Read the model definition and answer for the solid it produces. Units are mm, in the model's axes. Round coordinates to 2 decimals unless told otherwise and drop trailing zeros. Write each loop counter-clockwise with the first axis right and the second up, starting at its lowest first coordinate (ties: lowest second). Pieces come first, ordered by that corner, then holes. Notation, with made-up numbers: (50, -33) -> (106, -33) arc R8 cw to (106, -20) -> close; hole circle Ø7 at (24.25, 81). An arc over 180 degrees is marked (long way). Return JSON: item names as keys, results as strings. Group by question number.
(1) Straight lines are drawn through the part: line 1 (X direction, y = 16, z = 6); line 2 (Z direction, x = 29, y = 16.25); line 3 (Z direction, x = 6.5, y = 4). For each, find the intervals that lie inside material, in ascending order.
(2) A cutting plane is placed at D-D on y = 15.5. Give the vertices of the cut face in (x, z).
(3) The mould has two halves that part along Y. Classify faces 1 (the cylindrical face through (14.05, 13.7, 14.79)), 2 (the cylindrical face through (30.908, 11.154, 23.399)), 3 (the flat face through (17, 0, 15)): released by +Y, released by -Y, zero draft, split by the parting line, or undercut.
(4) A cutting plane is placed at A-A on x = 5. Give the vertices of the cut face in (y, z).
(5) A cutting plane is placed at C-C on x = 17. Give the vertices of the cut face in (y, z), then the cut area to 3 significant figures.
(6) A cutting plane is placed at B-B on z = 6. Give the vertices of the cut face in (x, y).
```python
from build123d import *

# Parameters (mm, degrees)
SKETCH1_W           = 34
SKETCH1_H           = 22
SKETCH1_R           = 4
BOSS_EXTRUDE1_DEPTH = 30
SKETCH2_R           = 2
CUT_EXTRUDE1_DEPTH  = 23


with BuildPart() as part:
    # Sketch1 → Boss-Extrude1 (new body)
    with BuildSketch(Plane.XY):
        with Locations((17, 11)):
            Rectangle(SKETCH1_W, SKETCH1_H)
        with Locations((17, 11)):
            Circle(SKETCH1_R, mode=Mode.SUBTRACT)
    extrude(amount=BOSS_EXTRUDE1_DEPTH)

    # Sketch2 → Cut-Extrude1 (cut, through all)
    with BuildSketch(Plane(origin=(0, 22, 0), x_dir=(1, 0, 0), z_dir=(0, 1, 0))):
        with Locations((5, -24)):
            Circle(SKETCH2_R)
        with Locations((5, -6)):
            Circle(SKETCH2_R)
        with Locations((29, -6)):
            Circle(SKETCH2_R)
        with Locations((29, -24)):
            Circle(SKETCH2_R)
    extrude(amount=-CUT_EXTRUDE1_DEPTH, mode=Mode.SUBTRACT)


solid = part.part
```
Checks:
{
 "1": {"line 1": "x = 0 to 3, 7 to 27, 31 to 34", "line 2": "z = 0 to 4, 8 to 22, 26 to 30", "line 3": "z = 0 to 4.68, 7.32 to 22.68, 25.32 to 30"},
 "2": {"outline": "(0, 0) -> (34, 0) -> (34, 30) -> (0, 30) -> close; hole circle Ø4 at (5, 6); hole circle Ø4 at (5, 24); hole circle Ø4 at (29, 6); hole circle Ø4 at (29, 24)"},
 "3": {"face 1": "undercut", "face 2": "zero draft", "face 3": "released by -Y"},
 "4": {"outline": "(0, 0) -> (22, 0) -> (22, 4) -> (0, 4) -> close; (0, 8) -> (22, 8) -> (22, 22) -> (0, 22) -> close; (0, 26) -> (22, 26) -> (22, 30) -> (0, 30) -> close"},
 "5": {"outline": "(0, 0) -> (7, 0) -> (7, 30) -> (0, 30) -> close; (15, 0) -> (22, 0) -> (22, 30) -> (15, 30) -> close", "area": "420 mm^2"},
 "6": {"outline": "(0, 0) -> (3, 0) -> (3, 22) -> (0, 22) -> close; (7, 0) -> (27, 0) -> (27, 22) -> (7, 22) -> close; (31, 0) -> (34, 0) -> (34, 22) -> (31, 22) -> close; hole circle Ø8 at (17, 11)"}
}
